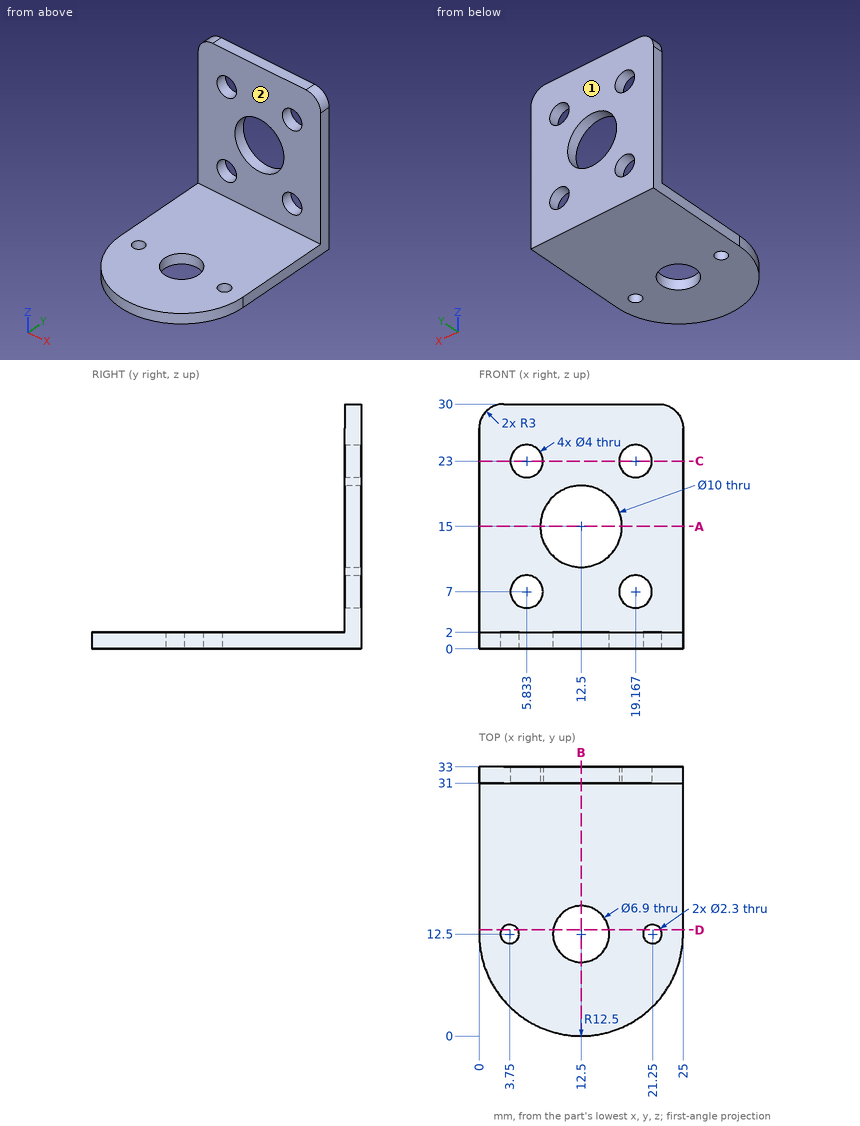
Can you work these out from the drawing? Everything is in mm from the part's minimum corner. A direction names the side the tool comes from. Round coordinates to 2 decimals unless told otherwise and drop trailing zeros. Order: outer loops, then holes, each group sorted by start corner. A loop starts at its lowest first (then second) coordinate and runs counter-clockwise, first axis right, second up. Notation, with made-up numbers: (14.25, 56.25) -> (62.25, 56.25) arc R24 ccw to (62.25, 76.25) -> close; hole circle Ø1 at (14, 24.25). An arc over 180 degrees is marked (long way). Use CSV: the item, a comma, the result in double quotes.
1. I want a section at A-A on z = 15. List the corners of the cut face in (x, y) for me.
Recorded:
outline,"(0, 31) -> (7.5, 31) -> (7.5, 33) -> (0, 33) -> close; (17.5, 31) -> (25, 31) -> (25, 33) -> (17.5, 33) -> close"
2. I want a section at D-D on y = 13. List the corners of the cut face in (x, z) for me (1 decimal).
Recorded:
outline,"(0, 0) -> (2.7, 0) -> (2.7, 2) -> (0, 2) -> close; (4.8, 0) -> (9.1, 0) -> (9.1, 2) -> (4.8, 2) -> close; (15.9, 0) -> (20.2, 0) -> (20.2, 2) -> (15.9, 2) -> close; (22.3, 0) -> (25, 0) -> (25, 2) -> (22.3, 2) -> close"
3. I want a section at C-C on z = 23. List the corners of the cut face in (x, y) for me, and give its area (3 significant figures).
Recorded:
outline,"(0, 31) -> (3.83, 31) -> (3.83, 33) -> (0, 33) -> close; (7.83, 31) -> (17.17, 31) -> (17.17, 33) -> (7.83, 33) -> close; (21.17, 31) -> (25, 31) -> (25, 33) -> (21.17, 33) -> close"
area,"34.0 mm2"
4. I'm going to push flat-ended pins straight in: P1, Ø6, axis at x = 12.5, z = 15, coming from the -Y side; P2, Ø6, axis at x = 17, z = 25, coming from the -Y side. Where does each tip first touch, or does it pass through?
Recorded:
P1,"passes through"
P2,"stops at y = 31"
5. Which directions (+Z, -Z, +X, -X, +Y, -Y) give clear straight access to the entire face, cutting with the end or side of a thin tool? Please do the marked faces 1 and 2.
Recorded:
face 1,"+Z, -Z, +X, -X, +Y"
face 2,"+Z, +X, -X, -Y"
6. I want a section at B-B on x = 12.5. List the corners of the cut face in (y, z) for me.
Recorded:
outline,"(0, 0) -> (9.05, 0) -> (9.05, 2) -> (0, 2) -> close; (15.95, 0) -> (33, 0) -> (33, 10) -> (31, 10) -> (31, 2) -> (15.95, 2) -> close; (31, 20) -> (33, 20) -> (33, 30) -> (31, 30) -> close"
7. I need wall thicknesses on line 1 along X through (y, z) = (32.4, 7); line 2 along Y through (x, z) = (15, 6.5); line 3 along Z through (x, y) = (1.75, 9.5). Which ranges of each line are inside material? Lowest first, please.
Recorded:
line 1,"x = 0 to 3.83, 7.83 to 17.17, 21.17 to 25"
line 2,"y = 31 to 33"
line 3,"z = 0 to 2"
